Part model, mm, in its own coordinate system. Give positions to 0.01 mm unless a question says otherwise; leave off trailing zeros. Order: outer loops, then holes, each group sorted by start corner. A loop starts at its lowest first (then second) coordinate and runs counter-clockwise, first axis right, second up. Notation, with made-up numbers: (24, 18.5) - (48, 18.5) arc R23 cw to (48, 53.5) - close; hole circle Ø11 at (81, 49). An arc over 180 degrees is marked (long way). One line per item, written item: value.
```python
from build123d import *

# Parameters (mm, degrees)
F1_DEPTH = 50.8
F2_R     = 12.7
F3_DEPTH = 50.8


with BuildPart() as f1:
    # F0 (on Top) → F1 (new body)
    with BuildSketch(Plane.XY):
        with BuildLine():
            Line((-101.6, 101.6), (-101.6, 0))
            Line((-101.6, 0), (-101.6, -101.6))
            Line((-101.6, -101.6), (101.6, -101.6))
            Line((101.6, -101.6), (101.6, 0))
            Line((101.6, 0), (101.6, 101.6))
            ThreePointArc((101.6, 101.6), (0, 127), (-101.6, 101.6))
        make_face()
    extrude(amount=F1_DEPTH)

    # F2 (on face) → F3 (cut)
    with BuildSketch(Plane.XY.offset(50.8)):
        with Locations((0, 63.5)):
            Circle(F2_R)
    extrude(amount=-F3_DEPTH, mode=Mode.SUBTRACT)


solid = f1.part
```
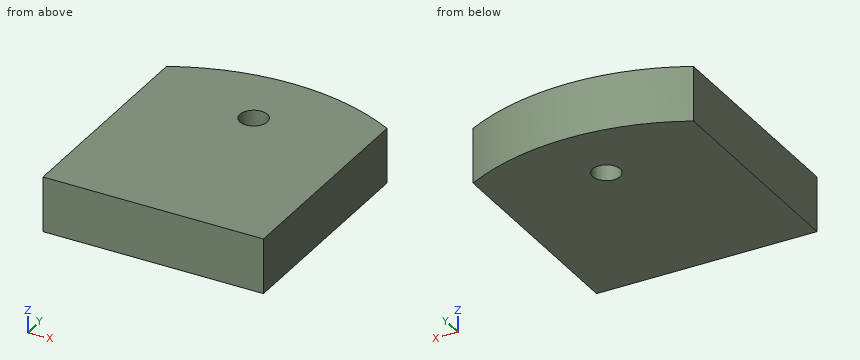
1) Pin check, flat tips, straight feed: pin 1 (3 mm diameter, centred on x = 69.5, z = 12, fed in from +Y); pin 2 (5 mm diameter, centred on x = 25, z = 29.5, fed in from +Y). Stop position of each tip, or through.
Outcome:
pin 1: stops at y = 116.01
pin 2: stops at y = 125.82
2) Cut at B-B, the plane y = 63.5. Give the cut face in (x, z), then the cut area to 3 significant figures.
Outcome:
outline: (-101.6, 0) - (-12.7, 0) - (-12.7, 50.8) - (-101.6, 50.8) - close; (12.7, 0) - (101.6, 0) - (101.6, 50.8) - (12.7, 50.8) - close
area: 9,030 mm^2
3) Cut at A-A, the plane x = 0. Give the cut face in (y, z).
Outcome:
outline: (-101.6, 0) - (50.8, 0) - (50.8, 50.8) - (-101.6, 50.8) - close; (76.2, 0) - (127, 0) - (127, 50.8) - (76.2, 50.8) - close
4) Cut at C-C, the plane z = 35. Give the cut face in (x, y).
Outcome:
outline: (-101.6, -101.6) - (101.6, -101.6) - (101.6, 101.6) arc R215.9 ccw to (-101.6, 101.6) - close; hole circle Ø25.4 at (0, 63.5)
5) Drill centre lines: line 1 along Y through (x, z) = (0, 18.5); line 2 along X through (y, z) = (63, 15); line 3 along X through (y, z) = (68.5, 11). Where is each one in solid material? Low to high. Write a range as from..to.
Outcome:
line 1: y = -101.6..50.8, 76.2..127
line 2: x = -101.6..-12.69, 12.69..101.6
line 3: x = -101.6..-11.67, 11.67..101.6
6) Cut at D-D, the plane x = 77. Give the cut face in (y, z).
Outcome:
outline: (-101.6, 0) - (112.8, 0) - (112.8, 50.8) - (-101.6, 50.8) - close
